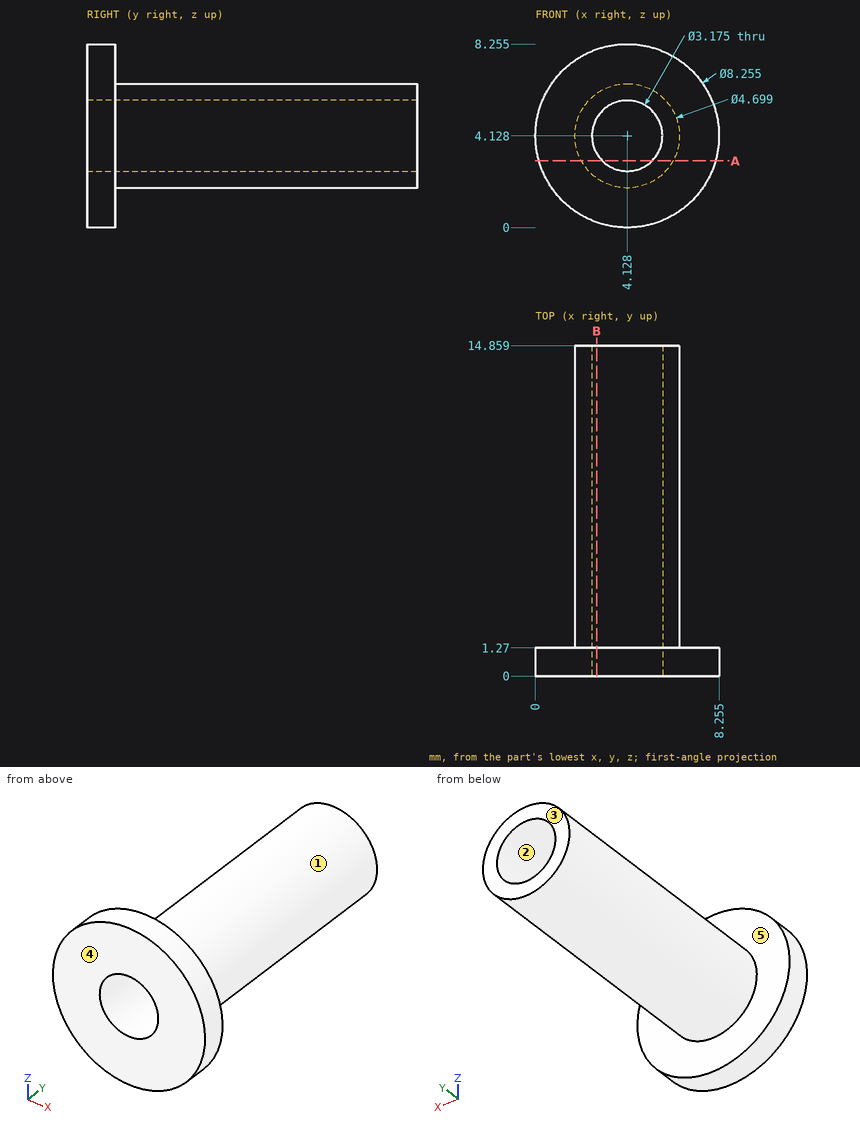
Could you check a few things on this drawing? It's one solid part, dimensions in mm from its lowest x, y, z. A direction names the side the tool comes from. Coordinates: 2 decimals unless noted, no trailing zeros. Order: outer loops, then holes, each group sorted by start corner. A loop starts at its lowest first (then second) coordinate and runs counter-clockwise, first axis right, second up.
1. For the marked faces 4 and 5, which set-ups out of +Z, -Z, +X, -X, +Y, -Y let a thin tool reach every point of the face, with its end or its side?
2. I'm going to push flat-ended pins straight in: pin 1 (4 mm diameter, centred on x = 1, y = 12, fed in from +Z); pin 2 (1.5 mm diameter, centred on x = 4.5, z = 3, fed in from -Y). Where does each tip first touch, or does it pass through?
3. If we section it at B-B (x = 2.75): Please give me the cut outline in (y, z) (1 decimal).
4. I need wall thicknesses on line 1 (Y direction, x = 3.5, z = 1.5); line 2 (X direction, y = 6, z = 5) (1 decimal); line 3 (X direction, y = 1.5, z = 5.5) (1 decimal). Which ranges of each line are inside material? Lowest first, please.
5. Thinking about a two-plate mould opening in X: for the marked faces 1, 2 and 3, which applies, +X half, -X half, draft (parallel to the pull), parting line (faces both ways), or undercut?
6. If we section it at A-A (z = 3): Please give me the cut outline in (x, y) (1 decimal).
Entries:
1. face 4: +Z, -Z, +X, -X, -Y
1. face 5: +Y
2. pin 1: stops at z = 6.19
2. pin 2: stops at y = 0
3. outline: (0, 0.2) - (1.3, 0.2) - (1.3, 2.2) - (14.9, 2.2) - (14.9, 3.3) - (0, 3.3) - close; (0, 4.9) - (14.9, 4.9) - (14.9, 6) - (1.3, 6) - (1.3, 8) - (0, 8) - close
4. line 1: y = 0 to 1.27
4. line 2: x = 1.9 to 2.8, 5.5 to 6.3
4. line 3: x = 2.2 to 3.3, 4.9 to 6
5. face 1: parting line
5. face 2: undercut
5. face 3: draft
6. outline: (0.2, 0) - (3, 0) - (3, 14.9) - (2.1, 14.9) - (2.1, 1.3) - (0.2, 1.3) - close; (5.2, 0) - (8.1, 0) - (8.1, 1.3) - (6.2, 1.3) - (6.2, 14.9) - (5.2, 14.9) - close
